from build123d import *

# Parameters (mm, degrees)
BOSS_EXTRU_1_DEPTH         = 5
ENL_V_MAT_EXTRU_2_DEPTH    = 5
R_P_TITION_LIN_AIRE1_COUNT = 3
R_P_TITION_LIN_AIRE1_PITCH = 123


with BuildPart() as part:
    # Esquisse1 → Boss.-Extru.1 (new body)
    with BuildSketch(Plane.XY):
        with BuildLine():
            Line((0, 0), (0, 21))
            ThreePointArc((0, 21), (0.878679656, 23.121320344), (3, 24))
            Line((3, 24), (199.45, 24))
            Line((199.45, 24), (199.45, 47))
            ThreePointArc((199.45, 47), (200.328679656, 49.121320344), (202.45, 50))
            Line((202.45, 50), (252.85, 50))
            ThreePointArc((252.85, 50), (254.971320344, 49.121320344), (255.85, 47))
            Line((255.85, 47), (255.85, 0))
            Line((255.85, 0), (245.85, 0))
            Line((245.85, 0), (245.85, 40))
            Line((245.85, 40), (209.45, 40))
            Line((209.45, 40), (209.45, 0))
            Line((209.45, 0), (173.45, 0))
            Line((173.45, 0), (173.45, 20))
            Line((173.45, 20), (137.05, 20))
            Line((137.05, 20), (137.05, 0))
            Line((137.05, 0), (101.05, 0))
            Line((101.05, 0), (101.05, 20))
            Line((101.05, 20), (64.65, 20))
            Line((64.65, 20), (64.65, 0))
            Line((64.65, 0), (46.4, 0))
            Line((46.4, 0), (46.4, 20))
            Line((46.4, 20), (10, 20))
            Line((10, 20), (10, 0))
            Line((10, 0), (0, 0))
        make_face()
    extrude(amount=BOSS_EXTRU_1_DEPTH)

    # Esquisse2 → Enlèv. mat.-Extru.2 (cut)
    with BuildSketch(Plane.XY.offset(5)):
        Polygon((6.5, 0), (6.5, 5), (8, 5), (8, 8), (6.5, 8), (6.5, 18), (3.5, 18), (3.5, 8), (2, 8), (2, 5), (3.5, 5), (3.5, 0), align=None)
    enl_v_mat_extru_2 = extrude(amount=-ENL_V_MAT_EXTRU_2_DEPTH, mode=Mode.SUBTRACT)

    # Répétition linéaire1: Enlèv. mat.-Extru.2 ×3
    with Locations(*[(i * R_P_TITION_LIN_AIRE1_PITCH, 0, 0) for i in range(1, R_P_TITION_LIN_AIRE1_COUNT)]):
        add(enl_v_mat_extru_2, mode=Mode.SUBTRACT)


solid = part.part
Verification items for the finished model (mm, model axes). A direction names the side the tool comes from. Coordinates: 2 decimals unless noted, no trailing zeros. Write each loop counter-clockwise with the first axis right and the second up, starting at its lowest first coordinate (ties: lowest second). Pieces come first, ordered by that corner, then holes. Notation, with made-up numbers: M 27,55 L 51,55 A21 ccw 51,70 Z; hole C 62,71.25 d10. An arc over 180 degrees is marked long. One line per question, with ' | ' between items.
1) Depth check by flat-ended pin: pin 1 Ø0.8 at (x, z) = (125.5, 2.5) entering from -Y; pin 2 Ø1.2 at (x, z) = (130.5, 2) entering from +Y; pin 3 Ø3 at (x, z) = (98, 3.5) entering from -Y. Enter the tip coordinate at first touch or a pass-through.
Solutions:
pin 1: y = 0 | pin 2: y = 24 | pin 3: y = 20
2) Sectioned sample at C-C on x = 216. Record the cut outline in (y, z), then the cut area to 3 significant figures.
Solutions:
outline: M 40,0 L 50,0 L 50,5 L 40,5 Z | area: 50.0 mm^2
3) Sectioned sample at A-A on y = 36.5. Record the cut outline in (x, z).
Solutions:
outline: M 199.45,0 L 209.45,0 L 209.45,5 L 199.45,5 Z; M 245.85,0 L 255.85,0 L 255.85,5 L 245.85,5 Z
4) Sectioned sample at D-D on x = 189. Record the cut outline in (y, z).
Solutions:
outline: M 0,0 L 24,0 L 24,5 L 0,5 Z
5) Release check for a two-part mould opening along X. For faces 1 (the face through (249.5, 3, 3)), 2 (the face through (56, 0, 2)) record: +X half, -X half, draft (parallel to the pull), parting line (faces both ways), or undercut.
Solutions:
face 1: undercut | face 2: draft
6) Material ranges on L1, parallel to X at y = 39.5, z = 4.3; L2, parallel to X at y = 19.5, z = 0.95; L3, parallel to X at y = 44, z = 4.55, recorded low to high.
Solutions:
L1: 199.45 to 209.45, 245.85 to 255.85 | L2: 0 to 10, 46.4 to 64.65, 101.05 to 137.05, 173.45 to 209.45, 245.85 to 255.85 | L3: 199.45 to 255.85
7) Access from +Z, -Z, +X, -X, +Y, -Y to the whole of each face (thin tool, end or side, straight path). Record for faces 3 (the face through (157, 21, 0)), 4 (the face through (126.5, 13, 3)), 5 (the face through (100, 24, 2)).
Solutions:
face 3: -Z, +X, -X, +Y, -Y | face 4: +Z, -Z, -Y | face 5: +Z, -Z, -X, +Y
8) Sectioned sample at B-B on y = 12.5. State how many separate pieces and enclosed holes the cut face has, then the cut area to 3 significant figures.
Solutions:
separate pieces: 8 | enclosed holes: 0 | area: 506 mm^2
